Build history of the part. All positions in model axes, mm. Give positions to 0.01 mm unless a question says otherwise; leave off trailing zeros. Loops run counter-clockwise (first coordinate to the right, second up) from the corner with the lowest first, then second, coordinate; pieces in that order, holes last. Notation, with made-up numbers: (-13.5, 14.5) -> (32.5, 14.5) arc R23 cw to (32.5, 22.5) -> close; hole circle Ø5 at (-10, -8). An arc over 180 degrees is marked (long way). Answer in a Markdown table with one row per item. Add a question column.
from build123d import *

# Parameters (mm, degrees)
SKETCH1_R           = 65
SKETCH1_R_2         = 50
BOSS_EXTRUDE1_DEPTH = 4.75
SKETCH2_R           = 1.5
CUT_EXTRUDE1_DEPTH  = 5
SKETCH3_R           = 1.5
CUT_EXTRUDE2_DEPTH  = 93.046523563


with BuildPart() as part:
    # Sketch1 → Boss-Extrude1 (new body)
    with BuildSketch(Plane(origin=(0, 0, 0), x_dir=(1, 0, 0), z_dir=(0, 1, 0))):
        with Locations(Location((0, 0, 0), (0, 0, 270))):
            Circle(SKETCH1_R)
        with Locations(Location((0, 0, 0), (0, 0, 270))):
            Circle(SKETCH1_R_2, mode=Mode.SUBTRACT)
    extrude(amount=BOSS_EXTRUDE1_DEPTH)

    # Sketch2 → Cut-Extrude1 (cut)
    with BuildSketch(Plane(origin=(0, 4.75, 0), x_dir=(1, 0, 0), z_dir=(0, 1, 0))):
        with Locations(Location((40.658639918, 40.658639918, 0), (0, 0, 270))):
            Circle(SKETCH2_R)
        with Locations(Location((40.658639918, -40.658639918, 0), (0, 0, 270))):
            Circle(SKETCH2_R)
        with Locations(Location((0, -57.5, 0), (0, 0, 270))):
            Circle(SKETCH2_R)
        with Locations(Location((-40.658639918, 40.658639918, 0), (0, 0, 270))):
            Circle(SKETCH2_R)
        with Locations(Location((0, 57.5, 0), (0, 0, 270))):
            Circle(SKETCH2_R)
        with Locations(Location((-40.658639918, -40.658639918, 0), (0, 0, 270))):
            Circle(SKETCH2_R)
    extrude(amount=-CUT_EXTRUDE1_DEPTH, mode=Mode.SUBTRACT)

    # Sketch3 → Cut-Extrude2 (cut, through all)
    with BuildSketch(Plane(origin=(0, 4.75, 0), x_dir=(1, 0, 0), z_dir=(0, 1, 0))):
        with Locations(Location((54.951905284, 9.5, 0), (0, 0, 270))):
            Circle(SKETCH3_R)
        with Locations(Location((-54.951905284, 9.5, 0), (0, 0, 90))):
            Circle(SKETCH3_R)
    extrude(amount=-CUT_EXTRUDE2_DEPTH, mode=Mode.SUBTRACT)


solid = part.part
(1) Wall check: line 1 along Z through (x, y) = (-42, 1.85); line 2 along X through (y, z) = (2, 0); line 3 along X through (y, z) = (2.7, 6). Give the ranges that are in metal, low to high. Write a range as from..to.
(2) Saw through at C-C, the plane x = -14. List the corners of the cut face in (y, z), then the cut area to 3 significant figures.
(3) Flat gauge pins, fed straight in: pin 1 Ø2 at (x, y) = (45, 4) entering from -Z; pin 2 Ø1.5 at (x, y) = (-45.5, 3) entering from +Z; pin 3 Ø1 at (y, z) = (2, -2.5) entering from -X. Where does each tip first touch, or does it go through?
(4) Saw through at D-D, the plane y = 3.3. State how many separate pieces and enclosed holes the cut face has, then the cut area to 3 significant figures.
(5) Saw through at B-B, the plane z = 0. List the corners of the cut face in (x, y).
(6) Two-plate mould, pull along X, no slides. Class faces 1 (the cylindrical face through (19.52, 2.34, 62)), 2 (the cylindrical face through (-39.64, 2.41, -41.76)), 3 (the flat face through (-38, 0, 33)): released by +X, released by -X, zero draft, split by the parting line, or undercut.
(7) Saw through at A-A, the plane x = 0. List the corners of the cut face in (y, z), then the cut area to 3 significant figures.
Worked answers:
| question | item | result |
|---|---|---|
| 1 | line 1 | -49.61..-41.33, -39.99..-27.13, 27.13..39.99, 41.33..49.61 |
| 1 | line 2 | -65..-50, 50..65 |
| 1 | line 3 | -64.72..-49.64, 49.64..64.72 |
| 2 | outline | (0, -63.47) -> (4.75, -63.47) -> (4.75, -48) -> (0, -48) -> close; (0, 48) -> (4.75, 48) -> (4.75, 63.47) -> (0, 63.47) -> close |
| 2 | area | 147 mm^2 |
| 3 | pin 1 | z = -47.84 |
| 3 | pin 2 | z = 47.14 |
| 3 | pin 3 | x = -64.97 |
| 4 | separate pieces | 1 |
| 4 | enclosed holes | 9 |
| 4 | area | 5,360 mm^2 |
| 5 | outline | (-65, 0) -> (-50, 0) -> (-50, 4.75) -> (-65, 4.75) -> close; (50, 0) -> (65, 0) -> (65, 4.75) -> (50, 4.75) -> close |
| 6 | face 1 | split by the parting line |
| 6 | face 2 | undercut |
| 6 | face 3 | zero draft |
| 7 | outline | (0, -65) -> (4.75, -65) -> (4.75, -59) -> (0, -59) -> close; (0, -56) -> (4.75, -56) -> (4.75, -50) -> (0, -50) -> close; (0, 50) -> (4.75, 50) -> (4.75, 56) -> (0, 56) -> close; (0, 59) -> (4.75, 59) -> (4.75, 65) -> (0, 65) -> close |
| 7 | area | 114 mm^2 |
